from build123d import *

# Parameters (mm, degrees)
ESQUISSE1_R                       = 3
BOSS_EXTRU_1_DEPTH                = 6
CHANFREIN1_SIZE                   = 0.5
DIAM_TRE_DU_PER_AGE_4_0_4_1_D     = 4
DIAM_TRE_DU_PER_AGE_4_0_4_1_DEPTH = 3.798278762
DIAM_TRE_DU_PER_AGE_4_0_4_1_TIP   = 1.201721238
BOSS_EXTRU_3_START                = -5
ESQUISSE2_R                       = 3
BOSS_EXTRU_3_DEPTH                = 5
DIAM_TRE_DU_PER_AGE_1_0_1_1_D     = 1
DIAM_TRE_DU_PER_AGE_1_0_1_1_DEPTH = 1.5
DIAM_TRE_DU_PER_AGE_1_0_1_1_TIP   = 0.30043031


with BuildPart() as part:
    # Esquisse1 → Boss.-Extru.1 (new body)
    with BuildSketch(Plane.XY):
        Circle(ESQUISSE1_R)
    extrude(amount=BOSS_EXTRU_1_DEPTH)

    # Chanfrein1
    chanfrein1_edges = [part.edges().sort_by_distance(p)[0] for p in [
        (-3, 0, 0),
    ]]
    chamfer(chanfrein1_edges, length=CHANFREIN1_SIZE)

    # Diamètre du perçage Ø4.0 (4)1
    with Locations(Plane.XY.offset(6)):
        with Locations((0, 0)):
            Hole(DIAM_TRE_DU_PER_AGE_4_0_4_1_D / 2, depth=DIAM_TRE_DU_PER_AGE_4_0_4_1_DEPTH)
            with Locations((0, 0, -(DIAM_TRE_DU_PER_AGE_4_0_4_1_DEPTH + DIAM_TRE_DU_PER_AGE_4_0_4_1_TIP / 2))):  # 118° drill point
                Cone(0, DIAM_TRE_DU_PER_AGE_4_0_4_1_D / 2, DIAM_TRE_DU_PER_AGE_4_0_4_1_TIP, mode=Mode.SUBTRACT)

    # Esquisse2 → Boss.-Extru.3 (add)
    with BuildSketch(Plane.XY.offset(6).offset(BOSS_EXTRU_3_START)):
        Circle(ESQUISSE2_R)
        Polygon((0, 2), (1.732050808, 1), (1.732050808, -1), (0, -2), (-1.732050808, -1), (-1.732050808, 1), align=None, mode=Mode.SUBTRACT)
    extrude(amount=BOSS_EXTRU_3_DEPTH)

    # Diamètre du perçage Ø1.0 (1)1
    with Locations(Plane(origin=(0, 0, 0), x_dir=(-1, 0, 0), z_dir=(0, 0, -1))):
        with Locations((0, 0)):
            Hole(DIAM_TRE_DU_PER_AGE_1_0_1_1_D / 2, depth=DIAM_TRE_DU_PER_AGE_1_0_1_1_DEPTH)
            with Locations((0, 0, -(DIAM_TRE_DU_PER_AGE_1_0_1_1_DEPTH + DIAM_TRE_DU_PER_AGE_1_0_1_1_TIP / 2))):  # 118° drill point
                Cone(0, DIAM_TRE_DU_PER_AGE_1_0_1_1_D / 2, DIAM_TRE_DU_PER_AGE_1_0_1_1_TIP, mode=Mode.SUBTRACT)


solid = part.part
Read the model definition and answer for the solid it produces. Units are mm, in the model's axes. A direction names the side the tool comes from. Coordinates: 2 decimals unless noted, no trailing zeros. Write each loop counter-clockwise with the first axis right and the second up, starting at its lowest first coordinate (ties: lowest second). Pieces come first, ordered by that corner, then holes. Notation, with made-up numbers: M 84,87 L 136,87 A16 cw 136,111 Z; hole C 44.25,-20 d1. An arc over 180 degrees is marked long. Use a Markdown table: item, result.
Q1. The part is cut by section B-B, the plane z = 5.05. Write down the section's boundary in (x, y), then the cut area to 3 significant figures.
Answer block:
| item | result |
|---|---|
| outline | C 0,0 d6; hole M -1.73,-1 L 0,-2 L 1.73,-1 L 1.73,1 L 0,2 L -1.73,1 Z |
| area | 17.9 mm2 |
Q2. The part is cut by section C-C, the plane z = 1.1. Write down the section's boundary in (x, y), then the cut area to 3 significant figures.
Answer block:
| item | result |
|---|---|
| outline | C 0,0 d6; hole C 0,0 d1 |
| area | 27.5 mm2 |
Q3. Straight lines are drawn through the part: L1, parallel to Y at x = 0, z = 0.7; L2, parallel to Y at x = 1.05, z = 3.35; L3, parallel to X at y = 0.15, z = 3.4. For each, find the intervals that lie inside material, in ascending order. Write a range as [from, to].
Answer block:
| item | result |
|---|---|
| L1 | y = [-3, -0.5], [0.5, 3] |
| L2 | y = [-2.81, -1.39], [1.39, 2.81] |
| L3 | x = [-3, -1.73], [1.73, 3] |
Q4. Which of the six approach directions +Z, -Z, +X, -X, +Y, -Y give full straight-line access (tool end or side, diameter ignored) to faces 4 (the face through (1, 0, 0)), 5 (the face through (-1.732, 0, 4))?
Answer block:
| item | result |
|---|---|
| face 4 | -Z, +X, -X, +Y, -Y |
| face 5 | +Z |
Q5. Each of these flat-tipped pins is pushed along its axis until it touches: pin 1 Ø1 at (x, z) = (1, 2.5) entering from +Y; pin 2 Ø1 at (y, z) = (-0.5, 3.5) entering from +X; pin 3 Ø0.6 at (y, z) = (-0.5, 3.5) entering from -X. Where does it stop, or does it pass through?
Answer block:
| item | result |
|---|---|
| pin 1 | stops at y = 2.96 |
| pin 2 | stops at x = 3 |
| pin 3 | stops at x = -2.99 |
Q6. Determine the mould class of faces 1 (the face through (-0.108, -0.488, 0.659)), 2 (the face through (-3, 0, 3)), 3 (the face through (2, 0, 6)) for opening direction X: released by +X, released by -X, zero draft, split by the parting line, or undercut.
Answer block:
| item | result |
|---|---|
| face 1 | undercut |
| face 2 | split by the parting line |
| face 3 | zero draft |
Q7. The part is cut by section A-A, the plane y = 0. Write down the section's boundary in (x, z), then the cut area to 3 significant figures.
Answer block:
| item | result |
|---|---|
| outline | M -3,0.5 L -2.5,0 L -0.5,0 L -0.5,1.3 L -1.73,2.04 L -1.73,6 L -3,6 Z; M 0.5,0 L 2.5,0 L 3,0.5 L 3,6 L 1.73,6 L 1.73,2.04 L 0.5,1.3 Z |
| area | 19.1 mm2 |
